Part model, mm, in its own coordinate system. Face numbers are marked on the shaded views. A direction names the side the tool comes from. Round coordinates to 2 decimals unless told otherwise and drop trailing zeros. Loops run counter-clockwise (first coordinate to the right, second up) from the corner with the lowest first, then second, coordinate; pieces in that order, holes last.
1) 3-axis set-ups, long thin cutter, end or side, ignore diameter. For the marked faces 1, 2 and 3: which of +Z, -Z, +X, -X, +Y, -Y reach the whole face in a straight line?
2) Probe line 1 (X direction, y = 0, z = 18); line 2 (Z direction, x = -23, y = -14). List the from-to ranges inside material, lowest first.
3) Band-saw the part on D-D, the plane z = 22.5. Write the cut outline in (x, y) (1 decimal).
4) Band-saw the part on B-B, the plane y = 17. Write the cut outline in (x, z).
5) Drop flat-ended pins along their axis: P1, Ø3, axis at y = -1.5, z = 10.5, coming from the -X side; P2, Ø8, axis at x = -0.5, z = 4, coming from the -Y side (3 decimals); P3, Ø1.6, axis at x = 0, y = 0, coming from the +Z side. Give the stop position or say it passes through.
6) Band-saw the part on A-A, the plane z = 16.75. Write the cut outline in (x, y) (1 decimal), then the cut area to 3 significant figures.
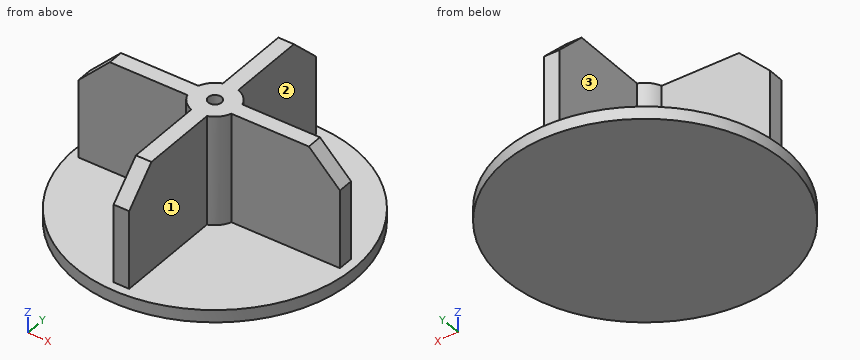
from build123d import *

# Parameters (mm, degrees)
F0_R     = 28.575
F1_DEPTH = 2.54
F3_DEPTH = 22.352
F4_SIZE  = 6.35
F5_R     = 4.7625
F6_DEPTH = 22.352
F8_D     = 2.7051
F8_DEPTH = 19.05
F8_TIP   = 0.8126940303


with BuildPart() as f1:
    # F0 (on Top) → F1 (new body)
    with BuildSketch(Plane.XY):
        Circle(F0_R)
    extrude(amount=F1_DEPTH)

    # F2 (on face) → F3 (join)
    with BuildSketch(Plane.XY.offset(2.54)):
        Polygon((26.67, -1.5875), (26.67, 1.5875), (1.5875, 1.5875), (1.5875, 26.67), (-1.5875, 26.67), (-1.5875, 1.5875), (-26.67, 1.5875), (-26.67, -1.5875), (-1.5875, -1.5875), (-1.5875, -26.67), (1.5875, -26.67), (1.5875, -1.5875), align=None)
    extrude(amount=F3_DEPTH)

    # F4
    f4_edges = [f1.edges().sort_by_distance(p)[0] for p in [
        (0, -26.67, 24.892),
        (26.67, 0, 24.892),
        (0, 26.67, 24.892),
        (-26.67, 0, 24.892),
    ]]
    chamfer(f4_edges, length=F4_SIZE)

    # F5 (on face) → F6 (join, through all)
    with BuildSketch(Plane.XY.offset(24.892)):
        Circle(F5_R)
    extrude(amount=-F6_DEPTH)

    # F8
    with Locations(Plane.XY.offset(24.892)):
        with Locations((0, 0)):
            Hole(F8_D / 2, depth=F8_DEPTH)
            with Locations((0, 0, -(F8_DEPTH + F8_TIP / 2))):  # 118° drill point
                Cone(0, F8_D / 2, F8_TIP, mode=Mode.SUBTRACT)


solid = f1.part
Reported:
1. face 1: +Z, +X, -Y
1. face 2: +Z, +X, +Y
1. face 3: +Z, -X, +Y
2. line 1: x = -26.67 to -1.35, 1.35 to 26.67
2. line 2: z = 0 to 2.54
3. outline: (-22.7, -1.6) - (-4.5, -1.6) arc R4.8 ccw to (-1.6, -4.5) - (-1.6, -22.7) - (1.6, -22.7) - (1.6, -4.5) arc R4.8 ccw to (4.5, -1.6) - (22.7, -1.6) - (22.7, 1.6) - (4.5, 1.6) arc R4.8 ccw to (1.6, 4.5) - (1.6, 22.7) - (-1.6, 22.7) - (-1.6, 4.5) arc R4.8 ccw to (-4.5, 1.6) - (-22.7, 1.6) - close; hole circle Ø2.7 at (0, 0)
4. outline: (-22.97, 0) - (22.97, 0) - (22.97, 2.54) - (1.59, 2.54) - (1.59, 24.89) - (-1.59, 24.89) - (-1.59, 2.54) - (-22.97, 2.54) - close
5. P1: stops at x = -26.67
5. P2: stops at y = -28.575
5. P3: stops at z = 5.51
6. outline: (-26.7, -1.6) - (-4.5, -1.6) arc R4.8 ccw to (-1.6, -4.5) - (-1.6, -26.7) - (1.6, -26.7) - (1.6, -4.5) arc R4.8 ccw to (4.5, -1.6) - (26.7, -1.6) - (26.7, 1.6) - (4.5, 1.6) arc R4.8 ccw to (1.6, 4.5) - (1.6, 26.7) - (-1.6, 26.7) - (-1.6, 4.5) arc R4.8 ccw to (-4.5, 1.6) - (-26.7, 1.6) - close; hole circle Ø2.7 at (0, 0)
6. area: 345 mm2
